Design review of the part built by this model. Coordinates are the model's own, in mm. A direction names the side the tool comes from. Give positions to 0.01 mm unless a question says otherwise; leave off trailing zeros. Loops run counter-clockwise (first coordinate to the right, second up) from the corner with the lowest first, then second, coordinate; pieces in that order, holes last.
from build123d import *

# Parameters (mm, degrees)
F1_DEPTH = 44.9
F2_T     = 10


# Not quite as in the source:
# - a shell that OpenCascade refuses in one call is made with other operations: the cavity is built on its own and cut out


with BuildPart() as f1:
    # F0 (on Front) → F1 (new body)
    with BuildSketch(Plane.XZ):
        with BuildLine():
            Line((-10.8614214341, 52.2791932931), (-55.5132357346, 20.2294568531))
            ThreePointArc((-55.5132357346, 20.2294568531), (-59.2261437786, 15.0907818347), (-59.1031517936, 8.7522851628))
            Line((-59.1031517936, 8.7522851628), (-41.1086877204, -41.8035860786))
            ThreePointArc((-41.1086877204, -41.8035860786), (-37.1445537144, -46.8302155121), (-30.9441109574, -48.4226575039))
            Line((-30.9441109574, -48.4226575039), (37.5255827113, -43.3174577507))
            ThreePointArc((37.5255827113, -43.3174577507), (43.3388920745, -40.8954764028), (46.5517141249, -35.4789891764))
            Line((46.5517141249, -35.4789891764), (54.1115878941, -0.8666353692))
            ThreePointArc((54.1115878941, -0.8666353692), (54.2619213312, 0.0049565354), (54.334653207, 0.886422737))
            Line((54.334653207, 0.886422737), (55.5578979933, 32.9868546181))
            ThreePointArc((55.5578979933, 32.9868546181), (53.4569722953, 39.5092382704), (47.6504120091, 43.1478142196))
            Line((47.6504120091, 43.1478142196), (-2.9450499877, 53.9354364594))
            ThreePointArc((-2.9450499877, 53.9354364594), (-7.0781470335, 53.9433412691), (-10.8614214341, 52.2791932931))
        make_face()
    extrude(amount=F1_DEPTH)

    # F2: shell of thickness 10, made by hand


with BuildPart() as f2_core1:
    # F2_t2: copy of F1
    add(f1.part)

    # the walls: a layer under each face that stays
    f2_faces = [f2_core1.faces().sort_by_distance(p)[0] for p in [
        (54.9462756001, -22.45, 16.9366386775),
        (22.3526810107, -22.45, 48.5416253395),
        (-33.1873285843, -22.45, 36.2543250731),
        (-50.105919757, -22.45, -16.5256504579),
        (3.2907358769, -22.45, -45.8700576273),
        (50.3316510095, -22.45, -18.1728122728),
        (-2.0584874118, 0, 2.8524646536),
    ]]
    thicken(f2_faces, amount=-F2_T, mode=Mode.SUBTRACT)


with BuildPart() as f1_1:
    add(f1.part)

    # what is left inside the walls is the cavity
    f2_cavity = [f2_core1.part.solids().sort_by_distance(p)[0] for p in [
        (-2.058487, -10.1, -10.915137),
    ]]
    add(f2_cavity, mode=Mode.SUBTRACT)


solid = f1_1.part
Q1. Draft analysis for pull direction X (two halves, no side actions). For faces 1 (the face through (-3, 0, 4)), 2 (the face through (44.945, -27.206, 17.093)), 3 (the face through (43.271, -22.136, -40.954)), state which applies: pulls with the +X half, pulls with the -X half, needs draft (parallel to the pull), parting line crosses it, or undercut.
Results:
face 1: needs draft
face 2: undercut
face 3: pulls with the +X half
Q2. Take a section at C-C (z = -18). Give the boundary of the cut face in (x, y), plus the area to 3 significant figures.
Results:
outline: (-49.58, -44.9) - (-38.97, -44.9) - (-38.97, -10) - (40.13, -10) - (40.13, -44.9) - (50.37, -44.9) - (50.37, 0) - (-49.58, 0) - close
area: 1,730 mm2
Q3. Tool access review of faces 4 (the face through (-40.81, -27.21, -12.82)), 5 (the face through (-59.199, -22.136, 15.177)): name each direction out of +Z, -Z, +X, -X, +Y, -Y from which nothing blocks a thin tool from reaching the whole face with its end or side.
Results:
face 4: -Y
face 5: -X, +Y, -Y
Q4. Take a section at A-A (y = -20.5). Give the boundary of the cut face in (x, z).
Results:
outline: (-59.1, 8.75) - (-41.11, -41.8) arc R10 ccw to (-30.94, -48.42) - (37.53, -43.32) arc R10 ccw to (46.55, -35.48) - (54.11, -0.87) arc R10 ccw to (54.33, 0.89) - (55.56, 32.99) arc R10 ccw to (47.65, 43.15) - (-2.95, 53.94) arc R10 ccw to (-10.86, 52.28) - (-55.51, 20.23) arc R10 ccw to start; hole (-49.68, 12.11) - (-31.69, -38.45) - (36.78, -33.35) - (44.34, 1.27) - (45.57, 33.37) - (-5.03, 44.16) - close
Q5. Insertion check: pin 1 (5 mm diameter, centred on x = -10.5, y = -18.5, fed in from +Z); pin 2 (3 mm diameter, centred on y = -10.5, z = -8.5, fed in from +X); pin 3 (6 mm diameter, centred on x = 33, y = -15.5, fed in from -Z); pin 4 (5 mm diameter, centred on x = 13, z = 3, fed in from +Y). Each pin has a flat end and moves straight along its axis. Give the tip position at first contact, or say it passes through.
Results:
pin 1: stops at z = 53.7
pin 2: stops at x = 52.77
pin 3: stops at z = -43.88
pin 4: stops at y = 0
Q6. Take a section at B-B (x = -24). Give the boundary of the cut face in (y, z), plus the area to 3 significant figures.
Results:
outline: (-44.9, -47.9) - (0, -47.9) - (0, 42.85) - (-44.9, 42.85) - (-44.9, 30.54) - (-10, 30.54) - (-10, -37.88) - (-44.9, -37.88) - close
area: 1,690 mm2
Q7. Wall thickness on line 1 (Y direction, x = -44.5, z = 3.5); line 2 (X direction, y = -20.5, z = 22); line 3 (X direction, y = -27.5, z = -7.5): over which ranges is each line inside the solid? List them lowest first.
Results:
line 1: y = -10 to 0
line 2: x = -53.05 to -35.9, 45.13 to 55.14
line 3: x = -53.32 to -42.7, 42.43 to 52.66
